Check sheet for the modelled part. Datum: model origin and axes. Units: mm. A direction names the side the tool comes from. Give positions to 0.01 mm unless a question says otherwise; leave off trailing zeros. Order: outer loops, then holes, each group sorted by start corner. A loop starts at its lowest first (then second) coordinate and runs counter-clockwise, first axis right, second up. Notation, with made-up numbers: (39.5, 1.5) - (73.5, 1.5) arc R21 cw to (73.5, 29.5) - close; hole circle Ø10 at (68, 1.5). An arc over 180 degrees is marked (long way). Answer in a Markdown table with one row per item.
from build123d import *

# Parameters (mm, degrees)
SKETCH1_R           = 20
BOSS_EXTRUDE1_DEPTH = 51
BOSS_EXTRUDE2_DEPTH = 10
BOSS_EXTRUDE3_DEPTH = 26
BOSS_EXTRUDE4_DEPTH = 10


with BuildPart() as part:
    # Sketch1 → Boss-Extrude1 (new body, symmetric)
    with BuildSketch(Plane(origin=(0, 0, 0), x_dir=(1, 0, 0), z_dir=(0, 1, 0))):
        Circle(SKETCH1_R)
    extrude(amount=BOSS_EXTRUDE1_DEPTH, both=True)

    # Sketch2 → Boss-Extrude2 (add)
    with BuildSketch(Plane(origin=(0, 51, 0), x_dir=(1, 0, 0), z_dir=(0, 1, 0))):
        with BuildLine():
            Line((15.889530325, 12.145897498), (-7.174782394, 42.319138828))
            ThreePointArc((-7.174782394, 42.319138828), (-26.567920967, 46.213928911), (-32.960703114, 27.495073445))
            Line((-32.960703114, 27.495073445), (-18.491697301, -7.619523011))
            ThreePointArc((-18.491697301, -7.619523011), (-9.967987772, 17.338950942), (15.889530325, 12.145897498))
        make_face()
    extrude(amount=-BOSS_EXTRUDE2_DEPTH)

    # Sketch2_3 → Boss-Extrude3 (add)
    with BuildSketch(Plane(origin=(0, 51, 0), x_dir=(1, 0, 0), z_dir=(0, 1, 0))):
        with BuildLine():
            ThreePointArc((-4.091930138, 33.209715704), (-4.883530929, 38.018186554), (-7.174782394, 42.319138828))
            ThreePointArc((-7.174782394, 42.319138828), (-26.567920967, 46.213928911), (-32.960703114, 27.495073445))
            ThreePointArc((-32.960703114, 27.495073445), (-16.179164668, 18.495239929), (-4.091930138, 33.209715704))
        make_face()
    extrude(amount=BOSS_EXTRUDE3_DEPTH)

    # Sketch3 → Boss-Extrude4 (add)
    with BuildSketch(Plane(origin=(0, 28, 0), x_dir=(-1, 0, 0), z_dir=(0, -1, 0))):
        with BuildLine():
            Line((18.491697301, -7.619523011), (20.177187538, -44.653612428))
            ThreePointArc((20.177187538, -44.653612428), (16.289787181, -53.030534966), (7.198092717, -54.650968393))
            Line((7.198092717, -54.650968393), (-38.995361437, -40.179987261))
            ThreePointArc((-38.995361437, -40.179987261), (-45.537524503, -33.661949585), (-43.950691193, -24.564330513))
            Line((-43.950691193, -24.564330513), (-15.889530325, 12.145897498))
            ThreePointArc((-15.889530325, 12.145897498), (-9.967987772, -17.338950942), (18.491697301, -7.619523011))
        make_face()
    extrude(amount=-BOSS_EXTRUDE4_DEPTH)


solid = part.part
(1) Thickness scan on L1, parallel to Y at x = -7, z = 48; L2, parallel to Y at x = -6.5, z = 0; L3, parallel to X at y = 1, z = -16.5. Record the ranges inside material, lowest first.
Geometry says:
| item | result |
|---|---|
| L1 | 28 to 38 |
| L2 | -51 to 51 |
| L3 | -11.3 to 11.3 |
(2) Cross-section at B-B, the plane x = 0. Record the cut outline in (y, z), then the cut area to 3 significant figures.
Geometry says:
| item | result |
|---|---|
| outline | (-51, -20) - (41, -20) - (41, -32.93) - (51, -32.93) - (51, 20) - (38, 20) - (38, 52.4) - (28, 52.4) - (28, 20) - (-51, 20) - close |
| area | 4,530 mm² |
(3) Cross-section at C-C, the plane y = 36. Record the cut outline in (x, z), then the cut area to 3 significant figures.
Geometry says:
| item | result |
|---|---|
| outline | (-20.18, 44.65) - (-18.49, 7.62) arc R20 ccw to (15.89, -12.15) - (43.95, 24.56) arc R10 ccw to (39, 40.18) - (-7.2, 54.65) arc R10 ccw to start |
| area | 3,480 mm² |
(4) Access from +Z, -Z, +X, -X, +Y, -Y to the whole of each face (thin tool, end or side, straight path). Record for faces 1 (the flat face through (-19.323, 32.93, 25.877)), 2 (the flat face through (-19, 77, -33)).
Geometry says:
| item | result |
|---|---|
| face 1 | -X, +Y, -Y |
| face 2 | +Z, -Z, +X, -X, +Y |
(5) Cross-section at D-D, the plane z = -3.5. Record the cut outline in (x, y).
Geometry says:
| item | result |
|---|---|
| outline | (-23.07, 41) - (-19.69, 41) - (-19.69, -51) - (19.69, -51) - (19.69, 28) - (22.5, 28) - (22.5, 38) - (19.69, 38) - (19.69, 51) - (-23.07, 51) - close |
(6) Cross-section at A-A, the plane z = 16. Record the cut outline in (x, y), then the cut area to 3 significant figures.
Geometry says:
| item | result |
|---|---|
| outline | (-18.87, 28) - (-12, 28) - (-12, -51) - (12, -51) - (12, 28) - (37.4, 28) - (37.4, 38) - (12, 38) - (12, 51) - (-12, 51) - (-12, 38) - (-18.87, 38) - close |
| area | 2,770 mm² |
(7) Gauge pin test, flat ends, axial feed: P1, Ø1, axis at x = 1.5, y = -32, coming from the +Z side (3 decimals); P2, Ø5, axis at x = 7.5, y = 13, coming from the +Z side; P3, Ø6, axis at x = 1, y = 30, coming from the +Z side. Record the tip position at first contact, or that the pin passes through.
Geometry says:
| item | result |
|---|---|
| P1 | z = 19.975 |
| P2 | z = 19.36 |
| P3 | z = 53.02 |
